from build123d import *

# Parameters (mm, degrees)
F0_W     = 177.8
F0_H     = 76.2
F1_DEPTH = 177.8
F2_W     = 50.8
F2_H     = 25.4
F3_DEPTH = 20.32
F4_W     = 2.5917394697
F4_H     = 7.6049772211
F5_DEPTH = 19.05


# Not quite as in the source:
# - a length typed as a fraction of an inch, garbled in the dataset ("3 / 203.2 mm" for 3/8 in), is restored


with BuildPart() as f1:
    # F0 (on Top) → F1 (new body)
    with BuildSketch(Plane.XY):
        with Locations((-17.2624356211, 54.5294494442)):
            Rectangle(F0_W, F0_H)
    extrude(amount=F1_DEPTH)

    # F2 (on face) → F3 (cut)
    with BuildSketch(Plane.XY.offset(177.8)):
        with Locations((-80.7624356211, 29.1294494442)):
            Rectangle(F2_W, F2_H)
        with Locations((46.2375643789, 29.1294494442)):
            Rectangle(F2_W, F2_H)
    extrude(amount=-F3_DEPTH, mode=Mode.SUBTRACT)

    # F4 (on face) → F5 (join)
    with BuildSketch(Plane.XY.offset(157.48)):
        with Locations((-82.0583053559, 29.7569380547)):
            Rectangle(F4_W, F4_H)
    extrude(amount=F5_DEPTH)

    # F7: F1 across plane


with BuildPart() as f1_1:
    add(f1.part)
    add(f1.part.mirror(Plane(origin=(-17.2624356211, 55.5353900382, 85.7815841584), x_dir=(0, -1, 0), z_dir=(-1, 0, 0))))


solid = f1_1.part
Can you work these out from the model? Positions are in its coordinate system, mm. A direction names the side the tool comes from. Round coordinates to 2 decimals unless told otherwise and drop trailing zeros. Loops run counter-clockwise (first coordinate to the right, second up) from the corner with the lowest first, then second, coordinate; pieces in that order, holes last. Notation, with made-up numbers: (44, 30) - (60, 30) arc R25 cw to (60, 69) - close; hole circle Ø9 at (-12.5, 8.25). An arc over 180 degrees is marked (long way). Write item = value, one per line. Start each with the question number.
(1) If we section it at A-A (z = 161): Please give me the cut outline in (x, y), and give its area (3 significant figures).
(2) If we section it at B-B (x = 43): Please give me the cut outline in (y, z).
(3) If I drill on probe 1 along Z at (x, y) = (36.5, 20.5); probe 2 along Y at (x, z) = (50.5, 165), over which ranges is the centre line in solid material (lowest first)? Write a range as [from, to].
(4) For faces 1 (the face through (20.838, 29, 168)), 2 (the face through (48.829, 30, 167)), 3 (the face through (-83.354, 30, 167)), which set-ups out of +Z, -Z, +X, -X, +Y, -Y let a thin tool reach every point of the face, with its end or its side?
(5) If we mould it in two halves opening along X, with no side actions, what happens to faces 4 (the face through (-81, 41.829, 168)), 5 (the face through (46.238, 30, 167)), 6 (the face through (-106.162, 54, 88))? For each: released by +X, released by -X, zero draft, split by the parting line, or undercut.
(6) For P1, Ø6, axis at y = 29, z = 171, coming from the +X side; P2, Ø0.8, axis at x = 47, y = 30.5, coming from the +Z side; P3, Ø7.5, axis at x = 35.5, y = 27, coming from the +Z side, each with a flat end and sliding along its axis, tell me the tip position at first contact or that it passes through.
Ans:
q1.outline = (-106.16, 41.83) - (-55.36, 41.83) - (-55.36, 16.43) - (20.84, 16.43) - (20.84, 41.83) - (71.64, 41.83) - (71.64, 92.63) - (-106.16, 92.63) - close; (-83.35, 25.95) - (-80.76, 25.95) - (-80.76, 33.56) - (-83.35, 33.56) - close; (46.24, 25.95) - (48.83, 25.95) - (48.83, 33.56) - (46.24, 33.56) - close
q1.area = 11,000 mm²
q2.outline = (16.43, 0) - (92.63, 0) - (92.63, 177.8) - (41.83, 177.8) - (41.83, 157.48) - (16.43, 157.48) - close
q3.probe_1 = [0, 157.48]
q3.probe_2 = [41.83, 92.63]
q4.face_1 = +Z, -Y
q4.face_2 = +Z, +X, -Y
q4.face_3 = +Z, -X, -Y
q5.face_4 = zero draft
q5.face_5 = undercut
q5.face_6 = released by -X
q6.P1 = 48.83
q6.P2 = 176.53
q6.P3 = 157.48
